For this review, use the dimensioned drawing (mm, ordinates from the lowest corner) and the shaded views. A direction names the side the tool comes from. Give positions to 0.01 mm unless a question says otherwise; leave off trailing zeros. Loops run counter-clockwise (first coordinate to the right, second up) from the corner with the lowest first, then second, coordinate; pieces in that order, holes last. Notation, with made-up numbers: M -14.75,22 L 28.25,22 A15 ccw 28.25,47 Z; hole C 88.5,-8.75 d9. An arc over 180 degrees is marked long. Return JSON: item names as keys, results as strings.
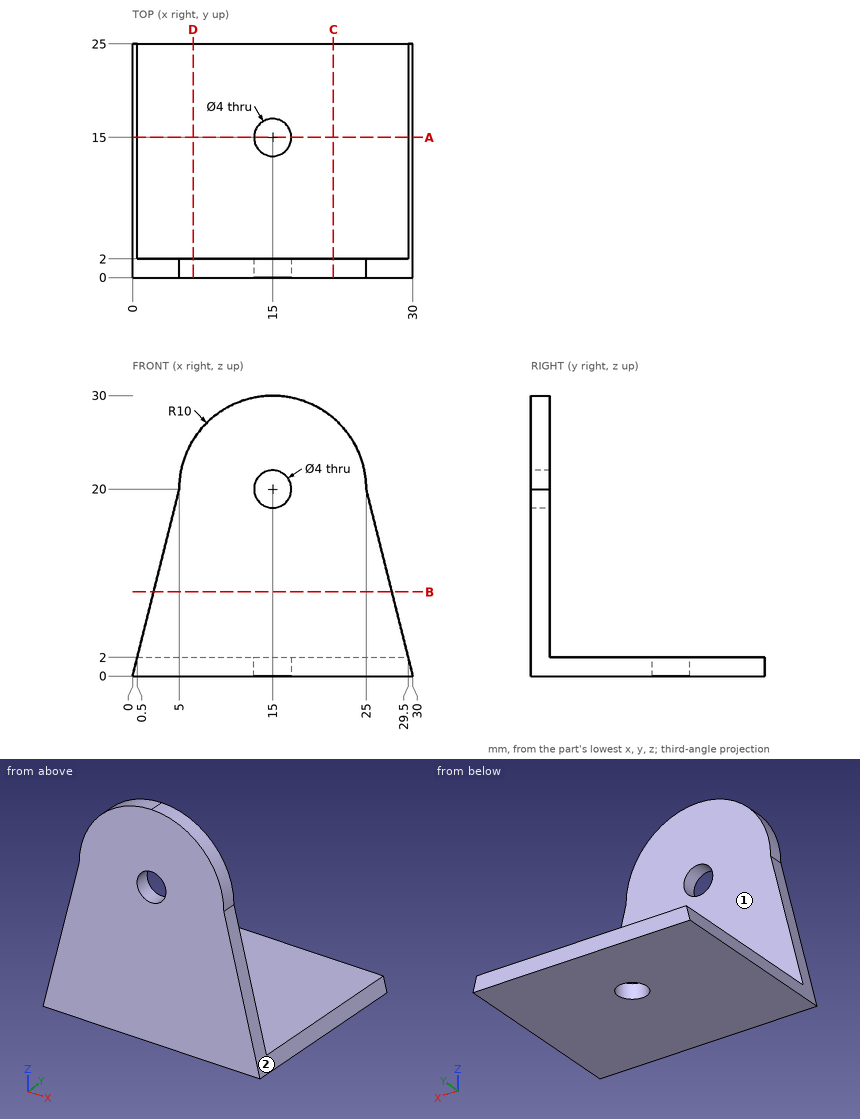
1) Consider section B-B on z = 9. Write out the cut boundary in (x, y), then the cut area to 3 significant figures.
From the geometry:
{"outline": "M 2.25,0 L 27.75,0 L 27.75,2 L 2.25,2 Z", "area": "51.0 mm²"}
2) Consider section A-A on y = 15. Write out the cut boundary in (x, z), then the cut area to 3 significant figures.
From the geometry:
{"outline": "M 0,0 L 13,0 L 13,2 L 0.5,2 Z; M 17,0 L 30,0 L 29.5,2 L 17,2 Z", "area": "51.0 mm²"}
3) Wall thickness on L1, parallel to X at y = 0.5, z = 20; L2, parallel to Y at x = 15, z = 1.1; L3, parallel to Z at x = 18.75, y = 15: over which ranges is each line inside the solid? List them lowest first. Write a range as from..to.
From the geometry:
{"L1": "5..13, 17..25", "L2": "0..13, 17..25", "L3": "0..2"}
4) Consider section C-C on x = 21.5. Write out the cut boundary in (y, z), then the cut area to 3 significant figures.
From the geometry:
{"outline": "M 0,0 L 25,0 L 25,2 L 2,2 L 2,27.6 L 0,27.6 Z", "area": "101 mm²"}
5) Tool access review of the marked faces 1 and 2: name each direction out of +Z, -Z, +X, -X, +Y, -Y from which nothing blocks a thin tool from reaching the whole face with its end or side.
From the geometry:
{"face 1": "+Z, +X, -X, +Y", "face 2": "+Z, +X, +Y, -Y"}
6) Consider section D-D on x = 6.5. Write out the cut boundary in (y, z).
From the geometry:
{"outline": "M 0,0 L 25,0 L 25,2 L 2,2 L 2,25.27 L 0,25.27 Z"}
7) Insertion check: pin 1 (1.5 mm diameter, centred on y = 3.5, z = 8.5, fed in from +X); pin 2 (10 mm diameter, centred on x = 13.5, y = 20.5, fed in from +Z); pin 3 (6 mm diameter, centred on x = 13.5, z = 7, fed in from +Y). Each pin has a flat end and moves straight along its axis. Give the tip position at first contact, or say it passes through.
From the geometry:
{"pin 1": "through", "pin 2": "z = 2", "pin 3": "y = 2"}
